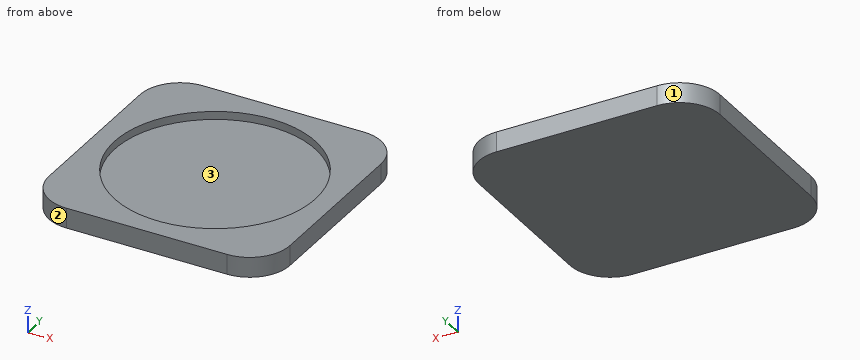
from build123d import *

# Parameters (mm, degrees)
F0_W     = 60
F0_H     = 60
F1_DEPTH = 5
F2_R     = 10
F3_R     = 25
F4_DEPTH = 2


with BuildPart() as f1:
    # F0 (on Top) → F1 (new body)
    with BuildSketch(Plane.XY):
        Rectangle(F0_W, F0_H)
    extrude(amount=F1_DEPTH)

    # F2
    f2_edges = [f1.edges().sort_by_distance(p)[0] for p in [
        (30, -30, 2.5),
        (30, 30, 2.5),
        (-30, -30, 2.5),
        (-30, 30, 2.5),
    ]]
    fillet(f2_edges, radius=F2_R)

    # F3 (on face) → F4 (cut)
    with BuildSketch(Plane.XY.offset(5)):
        Circle(F3_R)
    extrude(amount=-F4_DEPTH, mode=Mode.SUBTRACT)


solid = f1.part
Geometry: final body of the model. Coordinates: model frame, mm. Face numbers are marked on the shaded views. Coordinates: 2 decimals unless noted, no trailing zeros. Loops run counter-clockwise (first coordinate to the right, second up) from the corner with the lowest first, then second, coordinate; pieces in that order, holes last. Notation, with made-up numbers: M 7.5,11 L 40.5,11 A23 cw 40.5,35 Z; hole C 20,-1 d9. An arc over 180 degrees is marked long. One line per item, written item: value. Start each with the question number.
1) Material intervals for L1, parallel to X at y = -0.5, z = 4.15 (3 decimals); L2, parallel to Y at x = 0, z = 4.3; L3, parallel to Y at x = -15, z = 4.5, sorted ascending. Write a range as from..to.
2) Cut plane B-B (y = 0). Return loops of the section in (x, z), then the cut area to 3 significant figures.
3) Draft query along Y for the marked faces 1, 2 and 3. Return one class per face: released by +Y, released by -Y, zero draft, split by the parting line, or undercut.
4) Pin query (flat end, axial travel): P1, Ø3, axis at x = 7, y = -2.5, coming from the +Z side. Return the tip coordinate at first contact, or that it passes through.
5) Cut plane A-A (z = 2.25). Return loops of the section in (x, y), then the cut area to 3 significant figures.
Evaluation:
1. L1: -30..-24.995, 24.995..30
1. L2: -30..-25, 25..30
1. L3: -30..-20, 20..30
2. outline: M -30,0 L 30,0 L 30,5 L 25,5 L 25,3 L -25,3 L -25,5 L -30,5 Z
2. area: 200 mm^2
3. face 1: released by +Y
3. face 2: released by -Y
3. face 3: undercut
4. P1: z = 3
5. outline: M -30,-20 A10 ccw -20,-30 L 20,-30 A10 ccw 30,-20 L 30,20 A10 ccw 20,30 L -20,30 A10 ccw -30,20 Z
5. area: 3,510 mm^2
